Read the model definition and answer for the solid it produces. Units are mm, in the model's axes. A direction names the side the tool comes from. Coordinates: 2 decimals unless noted, no trailing zeros. Order: outer loops, then holes, each group sorted by start corner. A loop starts at its lowest first (then second) coordinate and runs counter-clockwise, first axis right, second up. Notation, with made-up numbers: (-17.5, -30) - (40.5, -30) arc R22 ccw to (40.5, -3) - close; hole circle Ø10 at (41, 81). An arc over 180 degrees is marked (long way). Write item = value, one per line.
from build123d import *

# Parameters (mm, degrees)
F0_R     = 6.5
F1_DEPTH = 5
F2_W     = 24
F2_H     = 5
F3_DEPTH = 50
F5_DEPTH = 5.001
F6_W     = 24
F6_H     = 5
F7_DEPTH = 5


with BuildPart() as f1:
    # F0 (on Top) → F1 (new body)
    with BuildSketch(Plane.XY):
        with BuildLine():
            Line((-12, 16), (-12, 0))
            ThreePointArc((-12, 0), (0, -12), (12, 0))
            Line((12, 0), (12, 16))
            Line((12, 16), (-12, 16))
        make_face()
        Circle(F0_R, mode=Mode.SUBTRACT)
    extrude(amount=F1_DEPTH)

    # F2 (on face) → F3 (join)
    with BuildSketch(Plane.XY.offset(5)):
        with Locations((0, 13.5)):
            Rectangle(F2_W, F2_H)
    extrude(amount=F3_DEPTH)

    # F4 (on face) → F5 (cut, through all)
    with BuildSketch(Plane.XZ.offset(-11)):
        with BuildLine():
            ThreePointArc((2, 41), (0, 43), (-2, 41))
            Line((-2, 41), (-2, 31))
            ThreePointArc((-2, 31), (0, 29), (2, 31))
            Line((2, 31), (2, 41))
        make_face()
    extrude(amount=-F5_DEPTH, mode=Mode.SUBTRACT)

    # F6 (on face) → F7 (join)
    with BuildSketch(Plane.XY.offset(55)):
        Polygon((23, 16), (12, 16), (12, 11), (-12, 11), (-12, -14), (23, -14), align=None)
        with Locations((0, 13.5)):
            Rectangle(F6_W, F6_H)
    extrude(amount=F7_DEPTH)


solid = f1.part
1) Flat-ended cylindrical pins translate along their axes: pin 1 Ø6 at (y, z) = (3, 6.5) entering from +X; pin 2 Ø1.5 at (x, z) = (-6, 52.5) entering from -Y; pin 3 Ø15 at (x, y) = (7.5, 5) entering from -Z. Find the tip coordinate at first contact, or state that the pin passes through.
Returned:
pin_1 = 12
pin_2 = 11
pin_3 = 0
2) The part is cut by section A-A (y = -7.5). Determine the outline of the cut face in (x, z), and give its area (3 significant figures).
Returned:
outline = (-12, 55) - (23, 55) - (23, 60) - (-12, 60) - close; (-9.37, 0) - (9.37, 0) - (9.37, 5) - (-9.37, 5) - close
area = 269 mm^2
3) Straight lines are drawn through the part: line 1 along Z through (x, y) = (-6, 5.75); line 2 along Y through (x, z) = (0, 2); line 3 along Z through (x, y) = (13, -7.5). For each, find the intervals that lie inside material, in ascending order. Write a range as from..to.
Returned:
line_1 = 0..5, 55..60
line_2 = -12..-6.5, 6.5..16
line_3 = 55..60
4) The part is cut by section B-B (x = 0). Determine the outline of the cut face in (y, z), and give its area (3 significant figures).
Returned:
outline = (-14, 55) - (11, 55) - (11, 43) - (16, 43) - (16, 60) - (-14, 60) - close; (-12, 0) - (-6.5, 0) - (-6.5, 5) - (-12, 5) - close; (6.5, 0) - (16, 0) - (16, 29) - (11, 29) - (11, 5) - (6.5, 5) - close
area = 405 mm^2
5) Determine the mould class of faces 5 (the face through (5, 1, 60)), 6 (the face through (0, 13, 43)), 7 (the face through (23, 1, 57)) for opening direction Z: pulls with the +Z half, pulls with the -Z half, needs draft (parallel to the pull), parting line crosses it, or undercut.
Returned:
face_5 = pulls with the +Z half
face_6 = undercut
face_7 = needs draft
6) The part is cut by section C-C (y = 1). Determine the outline of the cut face in (x, z).
Returned:
outline = (-12, 0) - (-6.42, 0) - (-6.42, 5) - (-12, 5) - close; (-12, 55) - (23, 55) - (23, 60) - (-12, 60) - close; (6.42, 0) - (12, 0) - (12, 5) - (6.42, 5) - close
7) The part is cut by section D-D (z = 11). Determine the outline of the cut face in (x, y), and give its area (3 significant figures).
Returned:
outline = (-12, 11) - (12, 11) - (12, 16) - (-12, 16) - close
area = 120 mm^2
8) For faces 1 (the face through (0, -12, 2)), 2 (the face through (2, 11, 30)), 3 (the face through (-2, 13, 36)), 4 (the face through (-5.158, -3.955, 2.465)), determine the directions among +Z, -Z, +X, -X, +Y, -Y from which every point of the face is accessible in a straight line to the end or side of a thin tool.
Returned:
face_1 = -Z, -Y
face_2 = +X, -X, -Y
face_3 = +Y, -Y
face_4 = -Z
